Can you work these out from the model? Positions are in its coordinate system, mm. Round coordinates to 2 decimals unless told otherwise and drop trailing zeros. Loops run counter-clockwise (first coordinate to the right, second up) from the corner with the lowest first, then second, coordinate; pieces in that order, holes last. Notation, with made-up numbers: (71, -2.5) -> (96, -2.5) arc R22 cw to (96, 14.5) -> close; hole circle Ø5 at (48.5, -11). An arc over 180 degrees is marked (long way). Use a Markdown table: item, result.
from build123d import *

# Parameters (mm, degrees)
SKETCH1_R           = 14.2875
SKETCH1_R_2         = 1.9939
BOSS_EXTRUDE1_DEPTH = 3.175


with BuildPart() as part:
    # Sketch1 → Boss-Extrude1 (new body)
    with BuildSketch(Plane.XY):
        with BuildLine():
            Line((0, 19.05), (25.4, 19.05))
            Line((25.4, 19.05), (50.8, 19.05))
            Line((50.8, 19.05), (50.8, -19.05))
            Line((50.8, -19.05), (25.4, -19.05))
            Line((25.4, -19.05), (0, -19.05))
            ThreePointArc((0, -19.05), (-19.05, 0), (0, 19.05))
        make_face()
        Circle(SKETCH1_R, mode=Mode.SUBTRACT)
        with Locations((38.1, -12.7)):
            Circle(SKETCH1_R_2, mode=Mode.SUBTRACT)
        with Locations((38.1, 0)):
            Circle(SKETCH1_R_2, mode=Mode.SUBTRACT)
        with Locations((38.1, 12.7)):
            Circle(SKETCH1_R_2, mode=Mode.SUBTRACT)
    extrude(amount=BOSS_EXTRUDE1_DEPTH)


solid = part.part
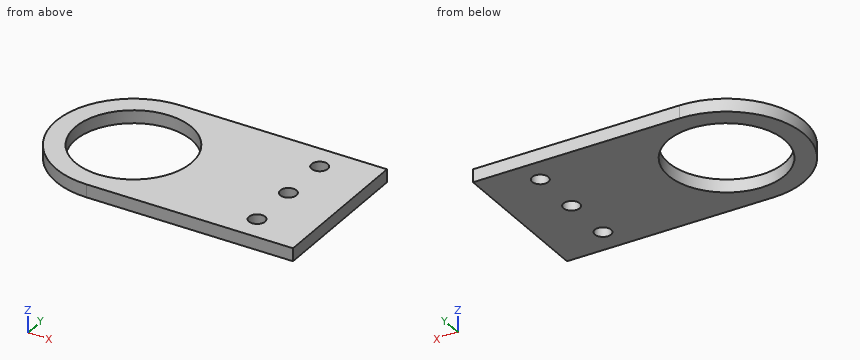
1. I want a section at D-D (x = 3.5). Please give me the cut outline in (y, z) (3 decimals).
Answer sheet:
| item | result |
|---|---|
| outline | (-19.05, 0) -> (-13.852, 0) -> (-13.852, 3.175) -> (-19.05, 3.175) -> close; (13.852, 0) -> (19.05, 0) -> (19.05, 3.175) -> (13.852, 3.175) -> close |
2. I need wall thicknesses on line 1 (Y direction, x = 38.1, z = 2.1); line 2 (X direction, y = 12.5, z = 2.55); line 3 (Y direction, x = -3, z = 1.1). Which ranges of each line are inside material? Lowest first, please.
Answer sheet:
| item | result |
|---|---|
| line 1 | y = -19.05 to -14.69, -10.71 to -1.99, 1.99 to 10.71, 14.69 to 19.05 |
| line 2 | x = -14.38 to -6.92, 6.92 to 36.12, 40.08 to 50.8 |
| line 3 | y = -18.81 to -13.97, 13.97 to 18.81 |
3. I want a section at B-B (x = 38.1). Please give me the cut outline in (y, z) (3 decimals).
Answer sheet:
| item | result |
|---|---|
| outline | (-19.05, 0) -> (-14.694, 0) -> (-14.694, 3.175) -> (-19.05, 3.175) -> close; (-10.706, 0) -> (-1.994, 0) -> (-1.994, 3.175) -> (-10.706, 3.175) -> close; (1.994, 0) -> (10.706, 0) -> (10.706, 3.175) -> (1.994, 3.175) -> close; (14.694, 0) -> (19.05, 0) -> (19.05, 3.175) -> (14.694, 3.175) -> close |
4. Will this pin go through, and if not, where does the flat tip stop? pin 1 Ø4.5 at (x, y) = (38.1, -12.7) entering from -Z.
Answer sheet:
| item | result |
|---|---|
| pin 1 | stops at z = 0 |
5. I want a section at A-A (y = 0). State how many separate pieces and enclosed holes the cut face has, plus the area to 3 significant figures.
Answer sheet:
| item | result |
|---|---|
| separate pieces | 3 |
| enclosed holes | 0 |
| area | 118 mm² |
